from build123d import *

# Parameters (mm, degrees)
SKETCH1_W               = 45
SKETCH1_H               = 50
CUT_EXTRUDE1_DEPTH      = 81.932070281
CUT_EXTRUDE1_DEPTH_BACK = 81.932070281
SKETCH2_W               = 10
SKETCH2_H               = 20
SHELL1_START            = 2.183039109
SHELL1_DEPTH            = 42.816960891
SHELL1_START_2          = 1.475e-06
SHELL1_2_DEPTH          = 10.999998525
SHELL1_START_3          = 41
SHELL1_3_DEPTH          = 4
SKETCH5_W               = 1
SKETCH5_H               = 1
SKETCH5_W_2             = 2
SKETCH5_H_2             = 2
SKETCH6_R               = 15
CUT_EXTRUDE4_DEPTH      = 1
SKETCH7_W               = 5
SKETCH7_H               = 25
BOSS_EXTRUDE1_DEPTH     = 30
CUT_EXTRUDE2_DEPTH      = 81.932070392
CUT_EXTRUDE2_DEPTH_BACK = 81.932070392
SKETCH3_R               = 7.5
FILLET1_R               = 5
SKETCH8_R               = 9
SKETCH8_R_2             = 7.5
BOSS_EXTRUDE2_DEPTH     = 2
FILLET2_R               = 5


with BuildPart() as part:
    # Sketch1 → Revolve1 (revolve)
    with BuildSketch(Plane.XY, mode=Mode.PRIVATE) as revolve1_sk:
        with Locations((22.5, 25)):
            Rectangle(SKETCH1_W, SKETCH1_H)
    revolve(revolve1_sk.sketch.rotate(Axis((0, 0, 0), (0, 1, 0)), 90), axis=Axis((0, 0, 0), (0, 1, 0)))

    # Sketch2 → Cut-Extrude1 (cut, two sides: drawn at the far end of the back side and taken through both)
    with BuildSketch(Plane.XY.offset(-CUT_EXTRUDE1_DEPTH_BACK)):
        with Locations((-43, 26)):
            Rectangle(SKETCH2_W, SKETCH2_H)
        with Locations((43, 26)):
            Rectangle(SKETCH2_W, SKETCH2_H)
        with BuildLine():
            Line((-45, 0), (-48, 0))
            Line((-48, 0), (-48, -7.78624056))
            Line((-48, -7.78624056), (48, -7.78624056))
            Line((48, -7.78624056), (48, 0))
            Line((48, 0), (45, 0))
            ThreePointArc((45, 0), (0, 10), (-45, 0))
        make_face()
    extrude(amount=CUT_EXTRUDE1_DEPTH + CUT_EXTRUDE1_DEPTH_BACK, mode=Mode.SUBTRACT)

    # Shell1: read off the stored shape, not the designer's step
    # Shell1 outline → Shell1 (cut)
    with BuildSketch(Plane(origin=(0, 0, 0), x_dir=(1, 0, 0), z_dir=(0, 1, 0)).offset(SHELL1_START)):
        with BuildLine():
            Line((33, -22.605309111), (33, 22.605309111))
            ThreePointArc((33, 22.605309111), (0, 40), (-33, 22.605309111))
            Line((-33, 22.605309111), (-33, -22.605309111))
            ThreePointArc((-33, -22.605309111), (0, -40), (33, -22.605309111))
        make_face()
    extrude(amount=SHELL1_DEPTH, mode=Mode.SUBTRACT)

    # Shell1 2 outline → Shell1 2 (cut)
    with BuildSketch(Plane(origin=(0, 0, 0), x_dir=(1, 0, 0), z_dir=(0, 1, 0)).offset(SHELL1_START_2)):
        with BuildLine():
            ThreePointArc((33, -22.605309111), (40, 0), (33, 22.605309111))
            Line((33, 22.605309111), (33, -22.605309111))
        make_face()
        with BuildLine():
            Line((-33, -22.605309111), (-33, 22.605309111))
            ThreePointArc((-33, 22.605309111), (-40, 0), (-33, -22.605309111))
        make_face()
    extrude(amount=SHELL1_2_DEPTH, mode=Mode.SUBTRACT)

    # Shell1 3 outline → Shell1 3 (cut)
    with BuildSketch(Plane(origin=(0, 0, 0), x_dir=(1, 0, 0), z_dir=(0, 1, 0)).offset(SHELL1_START_3)):
        with BuildLine():
            ThreePointArc((33, -22.605309111), (40, 0), (33, 22.605309111))
            Line((33, 22.605309111), (33, -22.605309111))
        make_face()
        with BuildLine():
            Line((-33, -22.605309111), (-33, 22.605309111))
            ThreePointArc((-33, 22.605309111), (-40, 0), (-33, -22.605309111))
        make_face()
    extrude(amount=SHELL1_3_DEPTH, mode=Mode.SUBTRACT)

    # Sketch5 → Cut-Revolve1 (revolve, cut)
    with BuildSketch(Plane.XY, mode=Mode.PRIVATE) as cut_revolve1_sk:
        with Locations((45, 46.5)):
            Rectangle(SKETCH5_W, SKETCH5_H)
        with Locations((45, 44.5)):
            Rectangle(SKETCH5_W, SKETCH5_H)
        with Locations((45, 40)):
            Rectangle(SKETCH5_W_2, SKETCH5_H_2)
    revolve(cut_revolve1_sk.sketch.rotate(Axis((0, 0, 0), (0, 1, 0)), 90), axis=Axis((0, 0, 0), (0, 1, 0)), mode=Mode.SUBTRACT)

    # Sketch6 → Cut-Extrude4 (cut)
    with BuildSketch(Plane(origin=(0, 50, 0), x_dir=(1, 0, 0), z_dir=(0, 1, 0))):
        with Locations(Location((-17.5, 17.5, 0), (0, 0, 270))):
            Circle(SKETCH6_R)
        with Locations(Location((17.5, 17.5, 0), (0, 0, 270))):
            Circle(SKETCH6_R)
        with Locations(Location((-17.5, -17.5, 0), (0, 0, 270))):
            Circle(SKETCH6_R)
        with Locations(Location((17.5, -17.5, 0), (0, 0, 270))):
            Circle(SKETCH6_R)
    extrude(amount=-CUT_EXTRUDE4_DEPTH, mode=Mode.SUBTRACT)

    # Sketch7 → Boss-Extrude1 (add)
    with BuildSketch(Plane.XZ.offset(-45)):
        with Locations((-10, 0)):
            Rectangle(SKETCH7_W, SKETCH7_H)
        with Locations((10, 0)):
            Rectangle(SKETCH7_W, SKETCH7_H)
    extrude(amount=BOSS_EXTRUDE1_DEPTH)

    # Sketch3 → Cut-Extrude2 (cut, two sides: drawn at the far end of the back side and taken through both)
    with BuildSketch(Plane(origin=(0, 0, 0), x_dir=(0, 0, -1), z_dir=(1, 0, 0)).offset(-CUT_EXTRUDE2_DEPTH_BACK)):
        with Locations((0, 26)):
            Circle(SKETCH3_R)
    extrude(amount=CUT_EXTRUDE2_DEPTH + CUT_EXTRUDE2_DEPTH_BACK, mode=Mode.SUBTRACT)

    # Fillet1
    fillet1_edges = [part.edges().sort_by_distance(p)[0] for p in [
        (-10, 15, -12.5),
        (-10, 15, 12.5),
        (10, 15, -12.5),
        (10, 15, 12.5),
    ]]
    fillet(fillet1_edges, radius=FILLET1_R)

    # Sketch8 → Boss-Extrude2 (add)
    with BuildSketch(Plane.ZY.offset(38)):
        with Locations(Location((0, 26, 0), (0, 0, 90))):
            Circle(SKETCH8_R)
        with Locations(Location((0, 26, 0), (0, 0, 180))):
            Circle(SKETCH8_R_2, mode=Mode.SUBTRACT)
    boss_extrude2 = extrude(amount=BOSS_EXTRUDE2_DEPTH)

    # Mirror1: Boss-Extrude2 across plane
    add(boss_extrude2.mirror(Plane(origin=(0, 0, 0), x_dir=(0, 0, 1), z_dir=(1, 0, 0))))

    # Fillet2
    fillet2_edges = [part.edges().sort_by_distance(p)[0] for p in [
        (-10, 45, -12.5),
        (-10, 45, 12.5),
        (10, 45, -12.5),
        (10, 45, 12.5),
    ]]
    fillet(fillet2_edges, radius=FILLET2_R)


solid = part.part
Build history of the part. All positions in model axes, mm. A direction names the side the tool comes from. Give positions to 0.01 mm unless a question says otherwise; leave off trailing zeros. Write each loop counter-clockwise with the first axis right and the second up, starting at its lowest first coordinate (ties: lowest second). Pieces come first, ordered by that corner, then holes. Notation, with made-up numbers: (-13, 43.5) - (35, 43.5) arc R20 ccw to (35, 76.5) - close; hole circle Ø4 at (-32.75, 73). An arc over 180 degrees is marked (long way). Use one line per item in the form item = value. Start each with the question number.
1. Band-saw the part on B-B on z = 0. Count the separate pieces of the cut face and the enclosed holes in it, plus the area to 3 significant figures.
2. 3-axis set-ups, long thin cutter, end or side, ignore diameter. For faces 1 (the face through (-17, 49, 17)), 2 (the face through (-9.96, 16.5, 11.07)), 3 (the face through (-40, 24, -7.4)), 4 (the face through (9.8, 39, 43.1)): which of +Z, -Z, +X, -X, +Y, -Y reach the whole face in a straight line?
3. Band-saw the part on A-A on y = 13. Write the cut outline in (x, z).
4. Probe line 1 (Y direction, x = -35, z = 0); line 2 (X direction, y = 18, z = -8.5); line 3 (Z direction, x = 10, y = 26). List the from-to ranges inside material, lowest first. Write a range as [from, to].
5. Two-plate mould, pull along Z, no slides. Class faces 5 (the face through (42.954, 40.014, 9.538)), 6 (the face through (10.04, 16.5, -11.07)), 7 (the face through (-10.2, 46, -43.5)): released by +Z, released by -Z, zero draft, split by the parting line, or undercut.
6. Drop flat-ended pins along their axis: pin 1 Ø4 at (x, z) = (-6, -6.5) entering from -Y; pin 2 Ø2.5 at (x, y) = (-11, 31) entering from +Z; pin 3 Ø12 at (x, y) = (-16.5, 30.5) entering from +Z. Give the stop position or say it passes through.
Conclusion:
q1.separate_pieces = 5
q1.enclosed_holes = 0
q1.area = 1,030 mm²
q2.face_1 = +Y
q2.face_2 = -Y
q2.face_3 = +Z, -Z, -X
q2.face_4 = none
q3.outline = circle Ø90 at (0, 0); hole (-33, -22.61) arc R40 ccw to (33, -22.61) - (33, 22.61) arc R40 ccw to (-33, 22.61) - close
q4.line_1 = [11, 18.5], [33.5, 41], [45, 50]
q4.line_2 = [-38, -33], [-12.5, -7.5], [7.5, 12.5], [33, 38]
q4.line_3 = [-43.87, -38.73], [-12.5, -7.5], [7.5, 12.5], [38.73, 43.87]
q5.face_5 = split by the parting line
q5.face_6 = undercut
q5.face_7 = zero draft
q6.pin_1 = 15
q6.pin_2 = 43.93
q6.pin_3 = 43.76
